```python
from build123d import *

# Parameters (mm, degrees)
BOSS_EXTRUDE1_DEPTH = 5
BOSS_EXTRUDE2_DEPTH = 25
FILLET1_R           = 10
CHAMFER3_SIZE       = 25
CHAMFER4_SIZE       = 15
SKETCH3_W           = 8
SKETCH3_H           = 42
CUT_EXTRUDE1_DEPTH  = 25
SKETCH4_W           = 8
SKETCH4_H           = 42
CUT_EXTRUDE2_DEPTH  = 25
FILLET2_R           = 10
SKETCH5_W           = 82
SKETCH5_H           = 4
CUT_EXTRUDE3_DEPTH  = 10
CHAMFER5_SIZE       = 10
CHAMFER6_SIZE       = 10


with BuildPart() as part:
    # Sketch1 → Boss-Extrude1 (new body)
    with BuildSketch(Plane.XY):
        Polygon((-167.5, -50), (167.5, -50), (167.5, 50), (41, 50), (41, -2), (-41, -2), (-41, 50), (-167.5, 50), align=None)
    extrude(amount=-BOSS_EXTRUDE1_DEPTH)

    # Sketch2 → Boss-Extrude2 (add)
    with BuildSketch(Plane(origin=(0, 0, -5), x_dir=(-1, 0, 0), z_dir=(0, 0, -1))):
        Polygon((-167.5, 50), (-162.5, 50), (-41, 50), (-41, 45), (-41, -2), (41, -2), (41, 45), (41, 50), (162.5, 50), (167.5, 50), (167.5, -50), (162.5, -50), (-162.5, -50), (-167.5, -50), align=None)
        Polygon((-162.5, 45), (-162.5, -45), (162.5, -45), (162.5, 45), (46, 45), (46, -7), (41, -7), (-41, -7), (-46, -7), (-46, 45), align=None, mode=Mode.SUBTRACT)
    extrude(amount=BOSS_EXTRUDE2_DEPTH)

    # Fillet1
    fillet1_edges = [part.edges().sort_by_distance(p)[0] for p in [
        (167.5, 50, -15),
        (167.5, -50, -15),
        (-167.5, -50, -15),
        (-167.5, 50, -15),
    ]]
    fillet(fillet1_edges, radius=FILLET1_R)

    # Chamfer3
    chamfer3_edges = [part.edges().sort_by_distance(p)[0] for p in [
        (-46, 19, -5),
        (46, 19, -5),
    ]]
    chamfer(chamfer3_edges, length=CHAMFER3_SIZE - 0.0001)  # a hair under: the kernel refuses the full size

    # Chamfer4
    chamfer4_edges = [part.edges().sort_by_distance(p)[0] for p in [
        (-41, 24, 0),
        (41, 24, 0),
    ]]
    chamfer(chamfer4_edges, length=CHAMFER4_SIZE)

    # Sketch3 → Cut-Extrude1 (cut)
    with BuildSketch(Plane(origin=(-41, 0, 0), x_dir=(0, 0, -1), z_dir=(1, 0, 0))):
        with Locations((26, 24)):
            Rectangle(SKETCH3_W, SKETCH3_H)
    extrude(amount=-CUT_EXTRUDE1_DEPTH, mode=Mode.SUBTRACT)

    # Sketch4 → Cut-Extrude2 (cut)
    with BuildSketch(Plane.ZY.offset(-41)):
        with Locations((-26, 24)):
            Rectangle(SKETCH4_W, SKETCH4_H)
    extrude(amount=-CUT_EXTRUDE2_DEPTH, mode=Mode.SUBTRACT)

    # Fillet2
    fillet2_edges = [part.edges().sort_by_distance(p)[0] for p in [
        (0, -2, 0),
        (-56, 24, 0),
        (56, 24, 0),
    ]]
    fillet(fillet2_edges, radius=FILLET2_R)

    # Sketch5 → Cut-Extrude3 (cut)
    with BuildSketch(Plane(origin=(0, -2, 0), x_dir=(1, 0, 0), z_dir=(0, 1, 0))):
        with Locations((0, 28)):
            Rectangle(SKETCH5_W, SKETCH5_H)
    extrude(amount=-CUT_EXTRUDE3_DEPTH, mode=Mode.SUBTRACT)

    # Chamfer5
    chamfer5_edges = [part.edges().sort_by_distance(p)[0] for p in [
        (162.5, 45, -17.5),
        (162.5, -45, -17.5),
        (-162.5, -45, -17.5),
        (-162.5, 45, -17.5),
    ]]
    chamfer(chamfer5_edges, length=CHAMFER5_SIZE)

    # Chamfer6
    chamfer6_edges = [part.edges().sort_by_distance(p)[0] for p in [
        (0, -7, -5),
    ]]
    chamfer(chamfer6_edges, length=CHAMFER6_SIZE)


solid = part.part
```
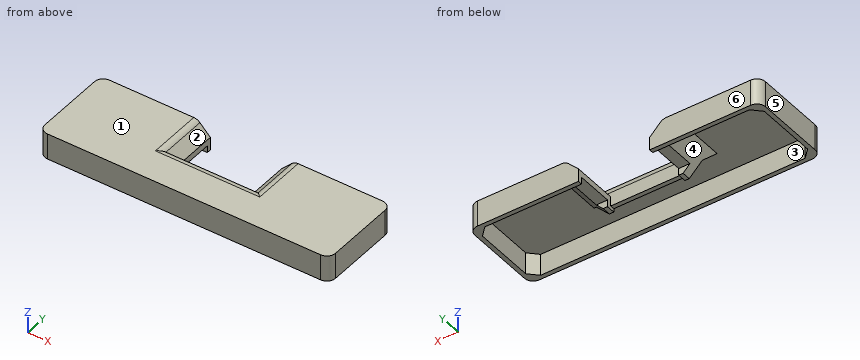
The model under review builds one solid part; all positions refer to its coordinate system, in mm. Face numbers are marked on the shaded views. A direction names the side the tool comes from. Round coordinates to 2 decimals unless told otherwise and drop trailing zeros. Write each loop counter-clockwise with the first axis right and the second up, starting at its lowest first coordinate (ties: lowest second). Pieces come first, ordered by that corner, then holes.
(1) Machinability: for the marked faces 1, 2 and 3, which of the approach directions +Z, -Z, +X, -X, +Y, -Y give a long, thin tool a straight path to every point of the face, cutting with its end or side? Answer none if there is none.
(2) Insertion check: pin 1 (8 mm diameter, centred on x = 81.5, y = 21.5, fed in from -Z); pin 2 (4 mm diameter, centred on x = -45, y = 20.5, fed in from -Z); pin 3 (2.5 mm diameter, centred on x = 11.5, y = -4.5, fed in from -Z). Each pin has a flat end and moves straight along its axis. Give the tip position at first contact, or say it passes through.
(3) Wall thickness on L1, parallel to Y at x = 136, z = -11.5; L2, parallel to X at y = -31, z = -10.75; L3, parallel to X at y = 26.5, z = -18.25: over which ranges is each line inside the solid? List them lowest first.
(4) We need section B-B on y = -22. Give the boundary of the cut face in (x, z).
(5) Mouldability with a two-part tool opening along X and no side actions: class the marked faces 4, 5 and 6 as +X half, -X half, draft (parallel to the pull), parting line (faces both ways), or undercut.
(6) We need section D-D on x = -16.5. Give the boundary of the cut face in (y, z), and give its area (3 significant figures).
(7) We need section A-A on y = 6.5. Give the boundary of the cut face in (x, z), and give its area (3 significant figures).
(8) We need section C-C on x = -105.5. Give the boundary of the cut face in (y, z).
Findings below:
1. face 1: +Z, +X, -X, +Y, -Y
1. face 2: +Z, +Y
1. face 3: -Z
2. pin 1: stops at z = -5
2. pin 2: stops at z = -22
2. pin 3: stops at z = -26
3. L1: y = -50 to -45, 45 to 50
3. L2: x = -167.5 to -162.5, 162.5 to 167.5
3. L3: x = -167.5 to -162.5, -57.75 to -41, 41 to 57.75, 162.5 to 167.5
4. outline: (-167.5, -30) - (-162.5, -30) - (-162.5, -5) - (162.5, -5) - (162.5, -30) - (167.5, -30) - (167.5, 0) - (-167.5, 0) - close
5. face 4: undercut
5. face 5: -X half
5. face 6: draft
6. outline: (-50, -30) - (-45, -30) - (-45, -5) - (-17, -5) - (-7, -15) - (-7, -26) - (-2, -26) - (-2, -10) arc R10 ccw to (-12, 0) - (-50, 0) - close
6. area: 499 mm2
7. outline: (-167.5, -30) - (-162.5, -30) - (-162.5, -5) - (-71, -5) - (-54, -22) - (-41, -22) - (-41, -15) - (-53.07, -2.93) arc R10 ccw to (-60.14, 0) - (-167.5, 0) - close; (41, -22) - (54, -22) - (71, -5) - (162.5, -5) - (162.5, -30) - (167.5, -30) - (167.5, 0) - (60.14, 0) arc R10 ccw to (53.07, -2.93) - (41, -15) - close
7. area: 2,020 mm2
8. outline: (-50, -30) - (-45, -30) - (-45, -5) - (45, -5) - (45, -30) - (50, -30) - (50, 0) - (-50, 0) - close
